```python
from build123d import *

# Parameters (mm, degrees)
SKETCH1_R           = 2.032
BOSS_EXTRUDE1_DEPTH = 2.54
BOSS_EXTRUDE2_DEPTH = 9.525


with BuildPart() as part:
    # Sketch1 → Boss-Extrude1 (new body)
    with BuildSketch(Plane(origin=(0, 0, 0), x_dir=(1, 0, 0), z_dir=(0, 1, 0))):
        with BuildLine():
            Line((-101.196460125, 62.269846472), (-107.93130861, -1.230153528))
            ThreePointArc((-107.93130861, -1.230153528), (-104.983139546, -10.325633674), (-96.249329296, -14.216651334))
            Line((-96.249329296, -14.216651334), (84.361550459, -14.216651334))
            ThreePointArc((84.361550459, -14.216651334), (93.095360709, -10.325633674), (96.043529773, -1.230153528))
            Line((96.043529773, -1.230153528), (89.308681288, 62.269846472))
            ThreePointArc((89.308681288, 62.269846472), (85.483184315, 69.764658916), (77.626701974, 72.778348666))
            Line((77.626701974, 72.778348666), (-89.514480811, 72.778348666))
            ThreePointArc((-89.514480811, 72.778348666), (-97.370963151, 69.764658916), (-101.196460125, 62.269846472))
        make_face()
        with Locations(Location((78.523810582, 59.410328666, 0), (0, 0, 270))):
            Circle(SKETCH1_R, mode=Mode.SUBTRACT)
        with Locations(Location((87.731310582, 2.260328666, 0), (0, 0, 270))):
            Circle(SKETCH1_R, mode=Mode.SUBTRACT)
        with Locations(Location((-5.943889418, 29.280848666, 0), (0, 0, 270))):
            Circle(SKETCH1_R, mode=Mode.SUBTRACT)
        with Locations(Location((-99.619089418, 2.260328666, 0), (0, 0, 270))):
            Circle(SKETCH1_R, mode=Mode.SUBTRACT)
        with Locations(Location((-90.411589418, 59.410328666, 0), (0, 0, 270))):
            Circle(SKETCH1_R, mode=Mode.SUBTRACT)
    extrude(amount=BOSS_EXTRUDE1_DEPTH)

    # Sketch4 → Boss-Extrude2 (add)
    with BuildSketch(Plane.XZ):
        with BuildLine():
            Line((99.200821479, 0.895289256), (92.465972995, -62.604710744))
            ThreePointArc((92.465972995, -62.604710744), (87.60655792, -72.125148173), (77.626701974, -75.953348666))
            Line((77.626701974, -75.953348666), (-89.514480811, -75.953348666))
            ThreePointArc((-89.514480811, -75.953348666), (-99.494336757, -72.125148173), (-104.353751831, -62.604710744))
            Line((-104.353751831, -62.604710744), (-111.088600316, 0.895289256))
            ThreePointArc((-111.088600316, 0.895289256), (-107.343628803, 12.44900728), (-96.249329296, 17.391651334))
            Line((-96.249329296, 17.391651334), (84.361550459, 17.391651334))
            ThreePointArc((84.361550459, 17.391651334), (95.455849966, 12.44900728), (99.200821479, 0.895289256))
        make_face()
        with BuildLine():
            ThreePointArc((-101.196460125, -62.269846472), (-97.370963151, -69.764658916), (-89.514480811, -72.778348666))
            Line((-89.514480811, -72.778348666), (77.626701974, -72.778348666))
            ThreePointArc((77.626701974, -72.778348666), (85.483184315, -69.764658916), (89.308681288, -62.269846472))
            Line((89.308681288, -62.269846472), (96.043529773, 1.230153528))
            ThreePointArc((96.043529773, 1.230153528), (93.095360709, 10.325633674), (84.361550459, 14.216651334))
            Line((84.361550459, 14.216651334), (-96.249329296, 14.216651334))
            ThreePointArc((-96.249329296, 14.216651334), (-104.983139546, 10.325633674), (-107.93130861, 1.230153528))
            Line((-107.93130861, 1.230153528), (-101.196460125, -62.269846472))
        make_face(mode=Mode.SUBTRACT)
    extrude(amount=-BOSS_EXTRUDE2_DEPTH)


solid = part.part
```
The listing builds one solid part. Answer for the finished solid, in the listing's coordinates (mm). A direction names the side the tool comes from. Round coordinates to 2 decimals unless told otherwise and drop trailing zeros. Loops run counter-clockwise (first coordinate to the right, second up) from the corner with the lowest first, then second, coordinate; pieces in that order, holes last.
1) Consider line 1 (Z direction, x = -76.5, y = 6.25); line 2 (X direction, y = 1.75, z = -59.5); line 3 (Y direction, x = -11, z = 5.5). Determine where each line is inside the solid, lowest interval first.
Outcome:
line 1: z = -75.95 to -72.78, 14.22 to 17.39
line 2: x = -104.68 to -92.44, -88.38 to 76.49, 80.55 to 92.8
line 3: y = 0 to 2.54
2) A cutting plane is placed at A-A on y = 5.75. Determine the outline of the cut face in (x, z) (1 decimal).
Outcome:
outline: (-111.1, 0.9) - (-104.4, -62.6) arc R14.9 ccw to (-89.5, -76) - (77.6, -76) arc R14.9 ccw to (92.5, -62.6) - (99.2, 0.9) arc R14.9 ccw to (84.4, 17.4) - (-96.2, 17.4) arc R14.9 ccw to start; hole (-107.9, 1.2) - (-101.2, -62.3) arc R11.7 ccw to (-89.5, -72.8) - (77.6, -72.8) arc R11.7 ccw to (89.3, -62.3) - (96, 1.2) arc R11.7 ccw to (84.4, 14.2) - (-96.2, 14.2) arc R11.7 ccw to start
3) A cutting plane is placed at C-C on z = -48.5. Determine the outline of the cut face in (x, y) (3 decimals), plus the area to 3 significant figures.
Outcome:
outline: (-105.85, 0) - (93.962, 0) - (93.962, 9.525) - (90.769, 9.525) - (90.769, 2.54) - (-102.657, 2.54) - (-102.657, 9.525) - (-105.85, 9.525) - close
area: 552 mm2
4) For faces 5 (the face through (-104.61, 5.98, -30.08)), 6 (the face through (-5.85, 1.25, -31.31)), determine the directions among +Z, -Z, +X, -X, +Y, -Y from which every point of the face is accessible in a straight line to the end or side of a thin tool.
Outcome:
face 5: +Y
face 6: +Y, -Y
5) A cutting plane is placed at B-B on x = 62. Determine the outline of the cut face in (y, z) (3 decimals), plus the area to 3 significant figures.
Outcome:
outline: (0, -75.953) - (9.525, -75.953) - (9.525, -72.778) - (2.54, -72.778) - (2.54, 14.217) - (9.525, 14.217) - (9.525, 17.392) - (0, 17.392) - close
area: 281 mm2
6) For a pull along Z with two mould halves and no side action, classify faces 1 (the face through (87.72, 4.7, -72.02)), 2 (the face through (-4, 0, -39)), 3 (the face through (85.393, 5.984, -69.845)), 4 (the face through (-92.395, 1.252, -59.851)) as released by +Z, released by -Z, zero draft, split by the parting line, or undercut.
Outcome:
face 1: released by -Z
face 2: zero draft
face 3: undercut
face 4: undercut
7) Given P1, Ø12, axis at x = -55.5, z = -27, coming from the +Y side; P2, Ø3.5, axis at x = 78.52, z = -59.41, coming from the -Y side; P3, Ø2, axis at x = -57.5, z = -39.5, coming from the -Y side; P4, Ø1.5, axis at y = 6, z = -32, coming from the -X side, each flat-ended and moving along its own axis, determine where each tip first touches the part or whether it passes through.
Outcome:
P1: stops at y = 2.54
P2: passes through
P3: stops at y = 0
P4: stops at x = -107.68
